```python
from build123d import *

# Parameters (mm, degrees)
F0_W     = 31.75
F0_H     = 50.8
F0_W_2   = 28.6004
F0_H_2   = 47.6504
F1_DEPTH = 101.6
F2_W     = 25.4
F2_H     = 25.4
F3_DEPTH = 50.801
F4_R     = 2.38125
F5_DEPTH = 31.751
F7_R     = 14.2875
F8_DEPTH = 31.751


with BuildPart() as f1:
    # F0 (on Top) → F1 (new body)
    with BuildSketch(Plane.XY):
        Rectangle(F0_W, F0_H)
        Rectangle(F0_W_2, F0_H_2, mode=Mode.SUBTRACT)
    extrude(amount=F1_DEPTH)

    # F2 (on face) → F3 (cut, through all)
    with BuildSketch(Plane.XZ.offset(25.4)):
        with Locations((0, 88.9)):
            Rectangle(F2_W, F2_H)
    extrude(amount=-F3_DEPTH, mode=Mode.SUBTRACT)

    # F4 (on face) → F5 (cut, through all)
    with BuildSketch(Plane(origin=(-15.875, 0, 0), x_dir=(0, -1, 0), z_dir=(-1, 0, 0))):
        with Locations((-9.332526, 85.532526)):
            Circle(F4_R)
        with Locations((9.332526, 85.532526)):
            Circle(F4_R)
    extrude(amount=-F5_DEPTH, mode=Mode.SUBTRACT)

    # F6: F1 across plane


with BuildPart() as f1_1:
    add(f1.part)
    add(f1.part.mirror(Plane.XY))

    # F7 (on face) → F8 (cut, through all)
    with BuildSketch(Plane(origin=(-15.875, 0, 0), x_dir=(0, -1, 0), z_dir=(-1, 0, 0))):
        Circle(F7_R)
    extrude(amount=-F8_DEPTH, mode=Mode.SUBTRACT)


solid = f1_1.part
```
Part model, mm, in its own coordinate system. A direction names the side the tool comes from. Round coordinates to 2 decimals unless told otherwise and drop trailing zeros. Loops run counter-clockwise (first coordinate to the right, second up) from the corner with the lowest first, then second, coordinate; pieces in that order, holes last.
Item 1: Cut at B-B, the plane y = 0. Give the cut face in (x, z) (1 decimal).
Item 2: Cut at A-A, the plane z = 0. Give the cut face in (x, y) (1 decimal), then the cut area to 3 significant figures.
Item 3: Drop flat-ended pins along their axis: P1, Ø1.7, axis at x = 1, y = -24.5, coming from the +Z side; P2, Ø4.5, axis at y = 9.33, z = 85.53, coming from the +X side; P3, Ø0.8, axis at x = 2.5, y = -24.5, coming from the -Z side. Give the stop position or say it passes through.
Item 4: Drill centre lines: line 1 (Y direction, x = 2, z = -68); line 2 (X direction, y = 10.5, z = 42) (3 decimals); line 3 (Z direction, x = -15.1, y = 0). Where is each one in solid material? Low to high.
Item 5: Cut at C-C, the plane x = 6. Give the cut face in (y, z), then the cut area to 3 significant figures.
Item 6: Mould opens along Y. For faces 1 (the face through (15.875, 17, 1)), 2 (the face through (15.08, 9.85, 83.21)), 3 (the face through (0, 25.4, 1)) say: +Y half, -Y half, draft (parallel to the pull), parting line (faces both ways), or undercut.
Item 7: Cut at D-D, the plane z = -70.5. Give the cut face in (x, y) (3 decimals).
Item 8: 3-axis set-ups, long thin cutter, end or side, ignore diameter. For faces 4 (the face through (-15.875, 17, 1)), 5 (the face through (0, 23.825, 1)): which of +Z, -Z, +X, -X, +Y, -Y reach the whole face in a straight line?
A:
1. outline: (-15.9, -101.6) - (-14.3, -101.6) - (-14.3, -14.3) - (-15.9, -14.3) - close; (-15.9, 14.3) - (-14.3, 14.3) - (-14.3, 101.6) - (-15.9, 101.6) - close; (14.3, -101.6) - (15.9, -101.6) - (15.9, -14.3) - (14.3, -14.3) - close; (14.3, 14.3) - (15.9, 14.3) - (15.9, 101.6) - (14.3, 101.6) - close
2. outline: (-15.9, -25.4) - (15.9, -25.4) - (15.9, -14.3) - (14.3, -14.3) - (14.3, -23.8) - (-14.3, -23.8) - (-14.3, -14.3) - (-15.9, -14.3) - close; (-15.9, 14.3) - (-14.3, 14.3) - (-14.3, 23.8) - (14.3, 23.8) - (14.3, 14.3) - (15.9, 14.3) - (15.9, 25.4) - (-15.9, 25.4) - close
2. area: 160 mm2
3. P1: stops at z = 76.2
3. P2: passes through
3. P3: stops at z = -76.2
4. line 1: y = -25.4 to -23.83, 23.83 to 25.4
4. line 2: x = -15.875 to -14.3, 14.3 to 15.875
4. line 3: z = -101.6 to -14.29, 14.29 to 101.6
5. outline: (-25.4, -76.2) - (-23.83, -76.2) - (-23.83, 76.2) - (-25.4, 76.2) - close; (23.83, -76.2) - (25.4, -76.2) - (25.4, 76.2) - (23.83, 76.2) - close
5. area: 480 mm2
6. face 1: draft
6. face 2: undercut
6. face 3: +Y half
7. outline: (-15.875, -25.4) - (15.875, -25.4) - (15.875, 25.4) - (-15.875, 25.4) - close; hole (-14.3, -23.825) - (14.3, -23.825) - (14.3, 23.825) - (-14.3, 23.825) - close
8. face 4: +Z, -Z, -X, +Y, -Y
8. face 5: +Z, -Z
